Design review of the part built by this model. Coordinates are the model's own, in mm. Face numbers are marked on the shaded views. A direction names the side the tool comes from. Coordinates: 2 decimals unless noted, no trailing zeros.
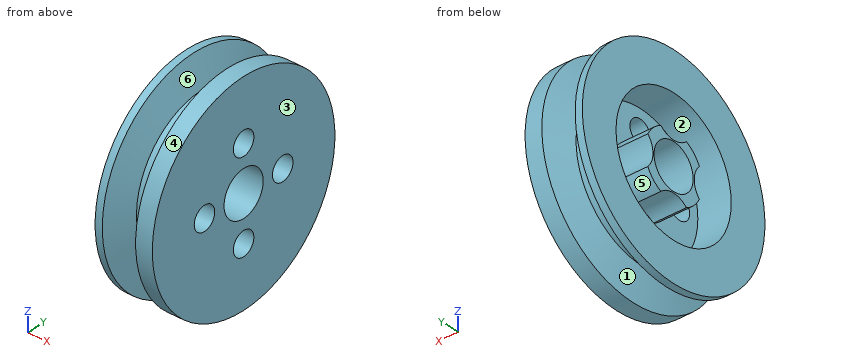
from build123d import *

# Parameters (mm, degrees)
F2_R           = 2.5
F2_R_2         = 4.7625
F3_DEPTH       = 10.001
F5_D           = 5
F5_CBORE_D     = 9
F5_CBORE_DEPTH = 7
F6_R           = 14.025
F6_R_2         = 7
F7_DEPTH       = 7
F8_DEPTH       = 2


with BuildPart() as f1:
    # F0 (on Front) → F1 (revolve)
    with BuildSketch(Plane.XZ):
        Polygon((0, 22.225), (0, 0), (10, 0), (10, 22.225), (8.4925, 22.225), (6.7910226281, 15.875), (3.2089773719, 15.875), (1.5075, 22.225), align=None)
    revolve(axis=Axis((5, 0, 0), (-1, 0, 0)))

    # F2 (on face) → F3 (cut, through all)
    with BuildSketch(Plane(origin=(0, 0, 0), x_dir=(0, -1, 0), z_dir=(-1, 0, 0))):
        with Locations((0, 9.525)):
            Circle(F2_R)
        with Locations((9.525, 0)):
            Circle(F2_R)
        with Locations((0, -9.525)):
            Circle(F2_R)
        with Locations((-9.525, 0)):
            Circle(F2_R)
        Circle(F2_R_2)
    extrude(amount=-F3_DEPTH, mode=Mode.SUBTRACT)

    # F5 (through all)
    with Locations(Plane(origin=(0, 0, 0), x_dir=(0, -1, 0), z_dir=(-1, 0, 0))):
        with Locations((0, 9.525), (-9.525, 0), (0, -9.525), (9.525, 0)):
            CounterBoreHole(F5_D / 2, F5_CBORE_D / 2, F5_CBORE_DEPTH)

    # F6 (on face) → F7 (cut)
    with BuildSketch(Plane(origin=(0, 0, 0), x_dir=(0, -1, 0), z_dir=(-1, 0, 0))):
        Circle(F6_R)
        Circle(F6_R_2, mode=Mode.SUBTRACT)
    extrude(amount=-F7_DEPTH, mode=Mode.SUBTRACT)

    # F8 (add): a face of the model
    f8_faces = [f1.faces().sort_by_distance(p)[0] for p in [
        (10, 0, -21.5963820715),
    ]]
    extrude(f8_faces, amount=F8_DEPTH)


solid = f1.part
1. For the marked faces 4, 5 and 6, list the 3-axis set-ups (+Z, -Z, +X, -X, +Y, -Y) from which the entire face can be reached by the end or side of a thin tool; tool diameter is ignored.
2. Mouldability with a two-part tool opening along Z and no side actions: class the marked faces 1, 2 and 3 as pulls with the +Z half, pulls with the -Z half, needs draft (parallel to the pull), parting line crosses it, or undercut.
3. To check wall thickness, follow line 1 (Y direction, x = 6.5, z = 6); line 2 (X direction, y = 2.5, z = 6); line 3 (X direction, y = 0, z = 20). State the ranges of each line that lie inside material, in increasing order.
4. Insertion check: pin 1 (1 mm diameter, centred on x = 8.5, y = 10, fed in from -Z); pin 2 (3 mm diameter, centred on x = 8, y = -13, fed in from +Z); pin 3 (1.5 mm diameter, centred on x = 4.5, y = -9.5, fed in from +Z). Each pin has a flat end and moves straight along its axis. Give the tip position at first contact, or say it passes through.
5. Add section A-A (y = 0). State how many separate pieces and enclosed holes the cut face has, and give its area (3 significant figures).
Solution:
1. face 4: +X, -X
1. face 5: -X
1. face 6: none
2. face 1: parting line crosses it
2. face 2: undercut
2. face 3: needs draft
3. line 1: y = -14.7 to -12.68, -3.61 to -2.8, 2.8 to 3.61, 12.68 to 14.7
3. line 2: x = 7 to 12
3. line 3: x = 0 to 2.1, 7.9 to 12
4. pin 1: stops at z = -20.09
4. pin 2: stops at z = 18.97
4. pin 3: stops at z = 13.25
5. separate pieces: 4
5. enclosed holes: 0
5. area: 176 mm2
